Can you work these out from the model? Positions are in its coordinate system, mm. Give positions to 0.01 mm unless a question says otherwise; leave off trailing zeros. Write each loop counter-clockwise with the first axis right and the second up, starting at its lowest first coordinate (ties: lowest second). Pieces come first, ordered by that corner, then holes.
Autodesk Inventor part; units mm, degrees
ref_plane "YZ Plane" through (0, 0, 0) normal (1, 0, 0) x (0, 1, 0)
ref_plane "XZ Plane" through (0, 0, 0) normal (0, 1, 0) x (-1, 0, 0)
ref_plane "XY Plane" through (0, 0, 0) normal (0, 0, 1) x (1, 0, 0)
sketch "草图1" plane through (0, 0, 0) normal (0, 0, 1) x (1, 0, 0)
  line L0 (-136.9893, 0) -> (-136.9893, 58)
  line L1 (-136.9893, 58) -> (-111.9893, 58)
  line L2 (-111.9893, 58) -> (-111.9893, 35)
  line L3 (-111.9893, 35) -> (-37.7393, 35)
  line L4 (-37.7393, 35) -> (-37.7393, 58)
  line L5 (-37.7393, 58) -> (-11.2393, 58)
  line L6 (-167.1393, 0) -> (43.9107, 0) construction
  line L7 (-11.2393, 58) -> (-11.2393, 40)
  line L8 (-11.2393, 40) -> (13.7607, 40)
  line L9 (13.7607, 40) -> (13.7607, 0)
  circle A0 centre (-108.9469, 0) radius 7.5
  line L10 (-136.9893, 0) -> (-136.9893, -58)
  line L11 (-136.9893, -58) -> (-111.9893, -58)
  line L12 (-111.9893, -58) -> (-111.9893, -35)
  line L13 (-111.9893, -35) -> (-37.7393, -35)
  line L14 (-37.7393, -35) -> (-37.7393, -58)
  line L15 (-37.7393, -58) -> (-11.2393, -58)
  line L16 (-11.2393, -58) -> (-11.2393, -40)
  line L17 (-11.2393, -40) -> (13.7607, -40)
  line L18 (13.7607, -40) -> (13.7607, 0)
  circle A1 centre (-58.7806, 0) radius 7.5
  point P0 (0, 0)
  point P1 (-131.9893, 53)
  point P2 (-115.9899, 52.8653)
  point P3 (-131.9893, 39)
  point P4 (-115.9893, 38.8653)
  point P5 (-124.4893, 22.14)
  point P6 (-41.9893, 22.14)
  point P7 (-31.2393, 18.5)
  point P8 (5.7607, 18.5)
  point P9 (-108.9469, 30)
  point P10 (-88.9469, 30)
  point P11 (-68.9469, 30)
  point P12 (-48.9469, 30)
  point P13 (-131.9893, 10)
  point P14 (-131.9893, -53)
  point P15 (-115.9899, -52.8653)
  point P16 (-131.9893, -39)
  point P17 (-115.9893, -38.8653)
  point P18 (-124.4893, -22.14)
  point P19 (-41.9893, -22.14)
  point P20 (-31.2393, -18.5)
  point P21 (5.7607, -18.5)
  point P22 (-108.9469, -30)
  point P23 (-88.9469, -30)
  point P24 (-68.9469, -30)
  point P25 (-48.9469, -30)
  point P26 (-131.9893, -10)
  point P27 (-7.5117, 35)
  point P28 (-7.5117, -35)
  dimension "d0" = 58
  dimension "d1" = 25
  dimension "d2" = 26.5
  dimension "d4" = 35
  dimension "d6" = 40
  dimension "d7" = 16
  dimension "d8" = 14
  dimension "d9" = 5
  dimension "d10" = 5
  dimension "d11" = 16
  dimension "d12" = 14
  dimension "d13" = 5
  dimension "d14" = 25
  dimension "d15" = 82.5
  dimension "d16" = 22.14
  dimension "d17" = 15
  dimension "d18" = 37
  dimension "d19" = 8
  dimension "d20" = 18.5
  dimension "d21" = 18.5
  dimension "d22" = 5
  dimension "d23" = 5
  dimension "d24" = 5
  dimension "d25" = 5
  dimension "d26" = 20
  dimension "d27" = 20
  dimension "d28" = 20
  dimension "d29" = 10
  dimension "d30" = 15
  dimension "d41" = 5
extrude "拉伸1" add sketch "草图1" along normal blind 4
hole "孔2" at (-131.9893, 53, 0) at (-115.9899, 52.8653, 0) at (-131.9893, 39, 0) at (-115.9893, 38.8653, 0) at (-124.4893, 22.14, 0) at (-41.9893, 22.14, 0) at (-31.2393, 18.5, 0) at (5.7607, 18.5, 0) at (-108.9469, 30, 0) at (-88.9469, 30, 0) at (-68.9469, 30, 0) at (-48.9469, 30, 0) at (-131.9893, 10, 0) at (-131.9893, -53, 0) at (-115.9899, -52.8653, 0) at (-115.9893, -38.8653, 0) at (-131.9893, -39, 0) at (-131.9893, -10, 0) at (-124.4893, -22.14, 0) at (-108.9469, -30, 0) at (-88.9469, -30, 0) at (-68.9469, -30, 0) at (-48.9469, -30, 0) at (5.7607, -18.5, 0) at (-31.2393, -18.5, 0) at (-41.9893, -22.14, 0) at (-7.5117, 35, 0) at (-7.5117, -35, 0) direction (0, 0, 1) diameter 3.2 end through all
sketch "草图2" plane through (0, 0, 4) normal (0, 0, 1) x (1, 0, 0)
  circle A0 centre (-7.5117, 35) radius 1.6 construction
  circle A1 centre (-31.2393, -18.5) radius 1.6 construction
  circle A2 centre (-48.9469, -30) radius 1.6 construction
  circle A3 centre (-88.9469, -30) radius 1.6 construction
  circle A4 centre (-124.4893, -22.14) radius 1.6 construction
  circle A5 centre (-131.9893, -39) radius 1.6 construction
  circle A6 centre (-115.9899, -52.8653) radius 1.6 construction
  circle A7 centre (-131.9893, 10) radius 1.6 construction
  circle A8 centre (-68.9469, 30) radius 1.6 construction
  circle A9 centre (-108.9469, 30) radius 1.6 construction
  circle A10 centre (-31.2393, 18.5) radius 1.6 construction
  circle A11 centre (-124.4893, 22.14) radius 1.6 construction
  circle A12 centre (-131.9893, 39) radius 1.6 construction
  circle A13 centre (-131.9893, 53) radius 1.6 construction
  circle A14 centre (-115.9899, 52.8653) radius 1.6 construction
  circle A15 centre (-115.9893, 38.8653) radius 1.6 construction
  circle A16 centre (-41.9893, 22.14) radius 1.6 construction
  circle A17 centre (5.7607, 18.5) radius 1.6 construction
  circle A18 centre (-88.9469, 30) radius 1.6 construction
  circle A19 centre (-48.9469, 30) radius 1.6 construction
  circle A20 centre (-131.9893, -53) radius 1.6 construction
  circle A21 centre (-115.9893, -38.8653) radius 1.6 construction
  circle A22 centre (-131.9893, -10) radius 1.6 construction
  circle A23 centre (-108.9469, -30) radius 1.6 construction
  circle A24 centre (-68.9469, -30) radius 1.6 construction
  circle A25 centre (5.7607, -18.5) radius 1.6 construction
  circle A26 centre (-41.9893, -22.14) radius 1.6 construction
  circle A27 centre (-7.5117, -35) radius 1.6 construction
  circle A28 centre (-58.7806, 0) radius 7.5 construction
  circle A29 centre (-108.9469, 0) radius 7.5 construction
  line L0 (-136.9893, 58) -> (-136.9893, -58) construction
  line L1 (-136.9893, -58) -> (-111.9893, -58) construction
  line L2 (-111.9893, -58) -> (-111.9893, -35) construction
  line L3 (-111.9893, -35) -> (-37.7393, -35) construction
  line L4 (-37.7393, -35) -> (-37.7393, -58) construction
  line L5 (-37.7393, -58) -> (-11.2393, -58) construction
  line L6 (-11.2393, -58) -> (-11.2393, -40) construction
  line L7 (-11.2393, -40) -> (13.7607, -40) construction
  line L8 (13.7607, -40) -> (13.7607, 40) construction
  line L9 (13.7607, 40) -> (-11.2393, 40) construction
  line L10 (-11.2393, 40) -> (-11.2393, 58) construction
  line L11 (-11.2393, 58) -> (-37.7393, 58) construction
  line L12 (-37.7393, 58) -> (-37.7393, 35) construction
  line L13 (-37.7393, 35) -> (-111.9893, 35) construction
  line L14 (-111.9893, 35) -> (-111.9893, 58) construction
  line L15 (-111.9893, 58) -> (-136.9893, 58) construction
  line L16 (0, 0) -> (-58.7806, 0) construction
  circle A30 centre (-131.9893, 39) radius 1.6
  circle A31 centre (-115.9899, 52.8653) radius 1.6
  point P0 (-32.1393, 38.9745)
  point P1 (-16.1393, 38.9745)
  point P2 (-16.1393, 52.9745)
  point P3 (-32.1393, 52.9745)
  point P4 (-32.1393, -38.9745)
  point P5 (-16.1393, -38.9745)
  point P6 (-16.1393, -52.9745)
  point P7 (-32.1393, -52.9745)
  dimension "d49" = 14
  dimension "d50" = 16
  dimension "d51" = 16
  dimension "d52" = 14
  dimension "d53" = 5.6
hole "孔4" at (-32.1393, 38.9745, 4) at (-16.1393, 38.9745, 4) at (-16.1393, 52.9745, 4) at (-32.1393, 52.9745, 4) at (-32.1393, -38.9745, 4) at (-16.1393, -38.9745, 4) at (-16.1393, -52.9745, 4) at (-32.1393, -52.9745, 4) at (-131.9893, -39, 4) at (-115.9893, -38.8653, 4) at (-131.9893, 39, 4) at (-115.9893, 38.8653, 4) at (-115.9899, 52.8653, 4) at (-131.9893, 53, 4) at (-131.9893, -53, 4) at (-115.9899, -52.8653, 4) direction (0, 0, -1) diameter 3.6 end through all
properties part number "130底盘5.0" material "尼龙 6/6"
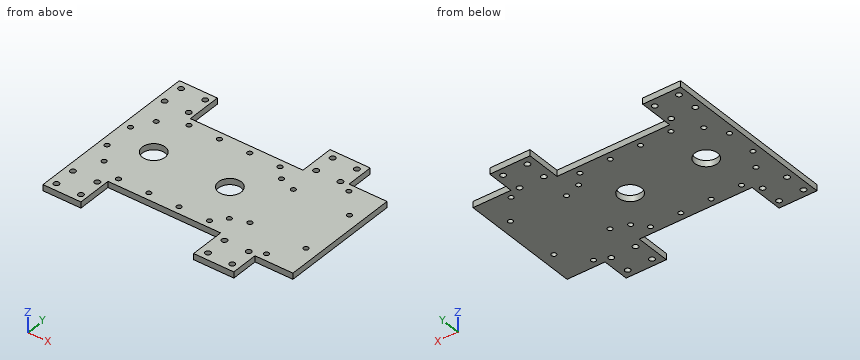
(1) Will these pins go through, and if not, where does the flat tip stop? P1, Ø2.5, axis at x = -31.24, y = -18.5, coming from the +Z side; P2, Ø2, axis at x = -56.5, z = 2, coming from the +Y side; P3, Ø2, axis at x = -94.5, z = 3, coming from the -Y side.
Returned:
P1: passes through
P2: stops at y = 35
P3: stops at y = -35
(2) Imagine slicing it at D-D, the plane y = 53. Write out the boundary of the cut face in (x, z), plus the area to 3 significant figures.
Returned:
outline: (-136.99, 0) - (-133.79, 0) - (-133.79, 4) - (-136.99, 4) - close; (-130.19, 0) - (-117.78, 0) - (-117.78, 4) - (-130.19, 4) - close; (-114.19, 0) - (-111.99, 0) - (-111.99, 4) - (-114.19, 4) - close; (-37.74, 0) - (-33.94, 0) - (-33.94, 4) - (-37.74, 4) - close; (-30.34, 0) - (-17.94, 0) - (-17.94, 4) - (-30.34, 4) - close; (-14.34, 0) - (-11.24, 0) - (-11.24, 4) - (-14.34, 4) - close
area: 148 mm2
(3) Imagine slicing it at C-C, the plane x = -103. Write out the boundary of the cut face in (y, z), plus the area to 3 significant figures.
Returned:
outline: (-35, 0) - (-4.57, 0) - (-4.57, 4) - (-35, 4) - close; (4.57, 0) - (35, 0) - (35, 4) - (4.57, 4) - close
area: 243 mm2
(4) Imagine slicing it at B-B, the plane y = 30. Write out the boundary of the cut face in (x, z), plus the area to 3 significant figures.
Returned:
outline: (-136.99, 0) - (-110.55, 0) - (-110.55, 4) - (-136.99, 4) - close; (-107.35, 0) - (-90.55, 0) - (-90.55, 4) - (-107.35, 4) - close; (-87.35, 0) - (-70.55, 0) - (-70.55, 4) - (-87.35, 4) - close; (-67.35, 0) - (-50.55, 0) - (-50.55, 4) - (-67.35, 4) - close; (-47.35, 0) - (13.76, 0) - (13.76, 4) - (-47.35, 4) - close
area: 552 mm2
(5) Imagine slicing it at A-A, the plane y = -10. Write out the boundary of the cut face in (x, z).
Returned:
outline: (-136.99, 0) - (-133.59, 0) - (-133.59, 4) - (-136.99, 4) - close; (-130.39, 0) - (13.76, 0) - (13.76, 4) - (-130.39, 4) - close
(6) If I drill on L1, parallel to X at y = -22, z = 0.25; L2, parallel to X at y = 30, z = 2.6; L3, parallel to X at y = 53, z = 2, over which ranges is the centre line in solid material (lowest first)?
Returned:
L1: x = -136.99 to -126.08, -122.9 to -43.58, -40.4 to 13.76
L2: x = -136.99 to -110.55, -107.35 to -90.55, -87.35 to -70.55, -67.35 to -50.55, -47.35 to 13.76
L3: x = -136.99 to -133.79, -130.19 to -117.78, -114.19 to -111.99, -37.74 to -33.94, -30.34 to -17.94, -14.34 to -11.24
